```python
from build123d import *

# Parameters (mm, degrees)
SKETCH1_W           = 32
SKETCH1_H           = 60
BOSS_EXTRUDE1_DEPTH = 5
SKETCH2_W           = 26
SKETCH2_H           = 54
CUT_EXTRUDE1_DEPTH  = 3
SKETCH6_W           = 20
SKETCH6_H           = 2
CUT_EXTRUDE4_DEPTH  = 2
SKETCH7_W           = 38
SKETCH7_H           = 66
BOSS_EXTRUDE3_DEPTH = 2
SKETCH4_W           = 8
SKETCH4_H           = 8
BOSS_EXTRUDE2_DEPTH = 1.5
SKETCH3_R           = 1.5
CUT_EXTRUDE2_DEPTH  = 5.5


with BuildPart() as part:
    # Sketch1 → Boss-Extrude1 (new body)
    with BuildSketch(Plane(origin=(0, 0, 0), x_dir=(1, 0, 0), z_dir=(0, 1, 0))):
        Rectangle(SKETCH1_W, SKETCH1_H)
    extrude(amount=BOSS_EXTRUDE1_DEPTH)

    # Sketch2 → Cut-Extrude1 (cut)
    with BuildSketch(Plane(origin=(0, 5, 0), x_dir=(1, 0, 0), z_dir=(0, 1, 0))):
        Rectangle(SKETCH2_W, SKETCH2_H)
    extrude(amount=-CUT_EXTRUDE1_DEPTH, mode=Mode.SUBTRACT)

    # Sketch6 → Cut-Extrude4 (cut)
    with BuildSketch(Plane(origin=(16, 0, -14), x_dir=(0, 0, 1), z_dir=(-1, 0, 0))):
        with Locations((14, 1)):
            Rectangle(SKETCH6_W, SKETCH6_H)
    cut_extrude4 = extrude(amount=CUT_EXTRUDE4_DEPTH, mode=Mode.SUBTRACT)

    # Sketch7 → Boss-Extrude3 (add)
    with BuildSketch(Plane.XZ):
        Rectangle(SKETCH7_W, SKETCH7_H)
    extrude(amount=BOSS_EXTRUDE3_DEPTH)

    # Sketch4 → Boss-Extrude2 (add)
    with BuildSketch(Plane(origin=(0, 2, 0), x_dir=(1, 0, 0), z_dir=(0, 1, 0))):
        with Locations((9, 23)):
            Rectangle(SKETCH4_W, SKETCH4_H)
        with Locations((-9, 23)):
            Rectangle(SKETCH4_W, SKETCH4_H)
        with Locations((9, -23)):
            Rectangle(SKETCH4_W, SKETCH4_H)
        with Locations((-9, -23)):
            Rectangle(SKETCH4_W, SKETCH4_H)
    extrude(amount=BOSS_EXTRUDE2_DEPTH)

    # Sketch3 → Cut-Extrude2 (cut)
    with BuildSketch(Plane(origin=(0, 3.5, 0), x_dir=(1, 0, 0), z_dir=(0, 1, 0))):
        with Locations(Location((-9.5, 23.5, 0), (0, 0, 270))):
            Circle(SKETCH3_R)
        with Locations(Location((9.5, 23.5, 0), (0, 0, 270))):
            Circle(SKETCH3_R)
        with Locations(Location((9.5, -23.5, 0), (0, 0, 270))):
            Circle(SKETCH3_R)
        with Locations(Location((-9.5, -23.5, 0), (0, 0, 270))):
            Circle(SKETCH3_R)
    extrude(amount=-CUT_EXTRUDE2_DEPTH, mode=Mode.SUBTRACT)

    # Mirror1: Cut-Extrude4 across plane
    add(cut_extrude4.mirror(Plane(origin=(0, 0, 0), x_dir=(0, 0, 1), z_dir=(1, 0, 0))), mode=Mode.SUBTRACT)


solid = part.part
```
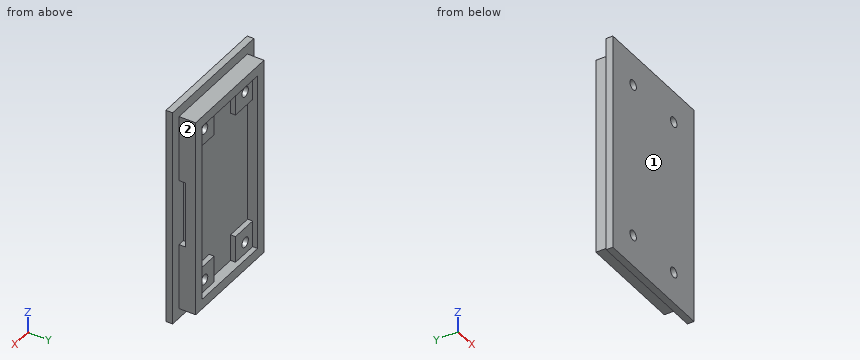
Part model, mm, in its own coordinate system. Face numbers are marked on the shaded views. A direction names the side the tool comes from. Coordinates: 2 decimals unless noted, no trailing zeros. Order: outer loops, then holes, each group sorted by start corner. A loop starts at its lowest first (then second) coordinate and runs counter-clockwise, first axis right, second up. Notation, with made-up numbers: (-37.5, 16.5) - (-9.5, 16.5) arc R36 ccw to (-9.5, 50.5) - close; hole circle Ø5 at (84, 70.25). An arc over 180 degrees is marked (long way). Return JSON: item names as keys, results as strings. Group by question number.
Item 1: Cut at B-B (x = -9.5). List the corners of the cut face in (y, z), plus the area to 3 significant figures.
Item 2: Cut at A-A (z = 23.5). List the corners of the cut face in (x, y), plus the area to 3 significant figures.
Item 3: Pin check, flat tips, straight feed: pin 1 (0.6 mm diameter, centred on x = 14.5, y = 1, fed in from -Z); pin 2 (0.8 mm diameter, centred on y = 3, z = -23.5, fed in from +X); pin 3 (0.6 mm diameter, centred on x = 14.5, y = 1.5, fed in from +Z). Stop position of each tip, or through.
Item 4: Cut at C-C (z = 0.5). List the corners of the cut face in (x, y), plus the area to 3 significant figures.
Item 5: Cut at D-D (x = -1.5). List the corners of the cut face in (y, z).
Item 6: Which spindle directions (+Z, -Z, +X, -X, +Y, -Y) get a long thin tool onto all of the face, cutting with end or side? Do the marked faces 1 and 2. Say none if no direction does.
Item 7: Drill centre lines: probe 1 along X at (y, z) = (1.9, -23.5); probe 2 along Y at (x, z) = (15, 3); probe 3 along Z at (x, y) = (7, 4.25). Where is each one in solid material? Low to high. Write a range as from..to.
Check values:
{
 "1": {"outline": "(-2, -33) - (0, -33) - (0, -30) - (5, -30) - (5, -27) - (3.5, -27) - (3.5, -25) - (-2, -25) - close; (-2, -22) - (3.5, -22) - (3.5, -19) - (2, -19) - (2, 19) - (3.5, 19) - (3.5, 22) - (-2, 22) - close; (-2, 25) - (3.5, 25) - (3.5, 27) - (5, 27) - (5, 30) - (0, 30) - (0, 33) - (-2, 33) - close", "area": "261 mm2"},
 "2": {"outline": "(-19, -2) - (-11, -2) - (-11, 3.5) - (-13, 3.5) - (-13, 5) - (-16, 5) - (-16, 0) - (-19, 0) - close; (-8, -2) - (8, -2) - (8, 3.5) - (5, 3.5) - (5, 2) - (-5, 2) - (-5, 3.5) - (-8, 3.5) - close; (11, -2) - (19, -2) - (19, 0) - (16, 0) - (16, 5) - (13, 5) - (13, 3.5) - (11, 3.5) - close", "area": "149 mm2"},
 "3": {"pin 1": "stops at z = -30", "pin 2": "stops at x = 16", "pin 3": "stops at z = 30"},
 "4": {"outline": "(-19, -2) - (19, -2) - (19, 0) - (14, 0) - (14, 2) - (16, 2) - (16, 5) - (13, 5) - (13, 2) - (-13, 2) - (-13, 5) - (-16, 5) - (-16, 2) - (-14, 2) - (-14, 0) - (-19, 0) - close", "area": "150 mm2"},
 "5": {"outline": "(-2, -33) - (0, -33) - (0, -30) - (5, -30) - (5, -27) - (2, -27) - (2, 27) - (5, 27) - (5, 30) - (0, 30) - (0, 33) - (-2, 33) - close"},
 "6": {"face 1": "+Z, -Z, +X, -X, -Y", "face 2": "+Z, -Z, +X, +Y"},
 "7": {"probe 1": "x = -16..-11, -8..8, 11..16", "probe 2": "y = -2..0, 2..5", "probe 3": "z = -30..-27, 27..30"}
}
